Source: CAD feature listing. Evaluate the final solid. Frame: model axes, mm. Face numbers are marked on the shaded views. A direction names the side the tool comes from. Give positions to 0.01 mm unless a question says otherwise; leave off trailing zeros. Loops run counter-clockwise (first coordinate to the right, second up) from the corner with the lowest first, then second, coordinate; pieces in that order, holes last. Notation, with made-up numbers: (51, 44) -> (81, 44) arc R35 ccw to (81, 79) -> close; hole circle Ø6 at (21.25, 1). An arc over 180 degrees is marked (long way). Answer as a JSON object with one key per item and string values. Group by question number.
from build123d import *

# Parameters (mm, degrees)
F0_R     = 12
F0_R_2   = 1.6
F1_DEPTH = 1.5
F2_DEPTH = 20
F3_R     = 1
F4_R     = 0.25


with BuildPart() as f1:
    # F0 (on Top) → F1 (new body)
    with BuildSketch(Plane.XY):
        Circle(F0_R)
        Circle(F0_R_2, mode=Mode.SUBTRACT)
    extrude(amount=F1_DEPTH)

    # F0 (on Top) → F2 (join)
    with BuildSketch(Plane.XY):
        Circle(F0_R_2)
    extrude(amount=F2_DEPTH)

    # F3
    f3_edges = [f1.edges().sort_by_distance(p)[0] for p in [
        (-12, 0, 1.5),
        (-1.6, 0, 1.5),
    ]]
    fillet(f3_edges, radius=F3_R)

    # F4
    f4_edges = [f1.edges().sort_by_distance(p)[0] for p in [
        (-1.6, 0, 20),
    ]]
    fillet(f4_edges, radius=F4_R)


solid = f1.part
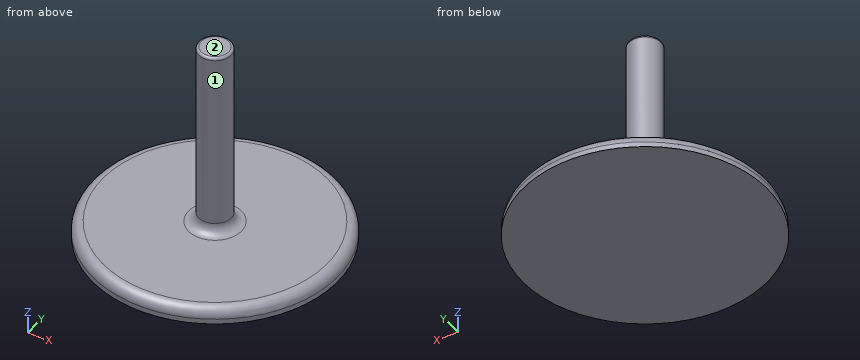
(1) First-contact query: pin 1 (2 mm diameter, centred on x = 0.5, z = 10.5, fed in from +Y); pin 2 (8 mm diameter, centred on x = 4.5, z = 4, fed in from +Y); pin 3 (4 mm diameter, centred on y = -1.5, z = 16.5, fed in from +X). Flat tips, straight axial feed; report the tip coordinate or a pass-through.
(2) Access query for the marked faces 1 and 2. Directions: +Z, -Z, +X, -X, +Y, -Y. A direction counts if a zero-diameter tool reaches every point of the face in a straight line with its end or side. Return the directions, or none.
(3) Section query C-C on z = 4. Return the cut outline in (x, y), plus the area to 3 significant figures.
(4) Section query A-A on x = 0. Return the cut outline in (y, z), plus the area to 3 significant figures.
(5) Material intervals for line 1 (Z direction, x = 2.5, y = 0.25); line 2 (Y direction, x = -0.5, z = 16); line 3 (X direction, y = 0.75, z = 4.5), sorted ascending. Write a range as from..to.
Result:
{
 "1": {"pin 1": "y = 1.6", "pin 2": "y = 11.77", "pin 3": "x = 1.6"},
 "2": {"face 1": "+Z", "face 2": "+Z, +X, -X, +Y, -Y"},
 "3": {"outline": "circle Ø3.2 at (0, 0)", "area": "8.04 mm²"},
 "4": {"outline": "(-12, 0) -> (12, 0) -> (12, 0.5) arc R1 ccw to (11, 1.5) -> (2.6, 1.5) arc R1 cw to (1.6, 2.5) -> (1.6, 19.75) arc R0.25 ccw to (1.35, 20) -> (-1.35, 20) arc R0.25 ccw to (-1.6, 19.75) -> (-1.6, 2.5) arc R1 cw to (-2.6, 1.5) -> (-11, 1.5) arc R1 ccw to (-12, 0.5) -> close", "area": "95.2 mm²"},
 "5": {"line 1": "0..1.5", "line 2": "-1.52..1.52", "line 3": "-1.41..1.41"}
}
